Here's how the part is built. I have some questions about the finished solid (model axes, mm). Give positions to 0.01 mm unless a question says otherwise; leave off trailing zeros. Order: outer loops, then holes, each group sorted by start corner. A loop starts at its lowest first (then second) coordinate and runs counter-clockwise, first axis right, second up. Notation, with made-up numbers: (56, 53) -> (105, 53) arc R10 ccw to (105, 60) -> close; hole circle Ø3 at (28.25, 89). An arc over 180 degrees is marked (long way). Write each question's results on one line, items separated by ' | '. Start each with the question number.
Q1. Imagine slicing it at D-D, the plane x = -51. Please give me the cut outline in (y, z).
Q2. Imagine slicing it at B-B, the plane y = 6.5. Please give me the cut outline in (x, z).
Q3. I'm going to push flat-ended pins straight in: pin 1 (3 mm diameter, centred on x = 68.5, y = -68.5, fed in from +Z); pin 2 (1.2 mm diameter, centred on y = -42.5, z = 2, fed in from -X). Where does each tip first touch, or does it pass through?
Q4. Imagine slicing it at C-C, the plane z = 0.85. Please give me the cut outline in (x, y).
Q5. Imagine slicing it at A-A, the plane x = -68.5. Please give me the cut outline in (y, z).
Q6. I need wall thicknesses on line 1 along Y through (x, z) = (68.5, 2); line 2 along Y through (x, z) = (-3.5, 1.45); line 3 along X through (y, z) = (-68.5, 2). Which ranges of each line are inside material? Lowest first, please. Write a range as [from, to].
```python
from build123d import *

# Parameters (mm, degrees)
F1_DEPTH = 2.5
F2_R     = 1.75
F3_DEPTH = 3.5
F4_DEPTH = 1
F5_R     = 1


with BuildPart() as f1:
    # F0 (on Top) → F1 (new body)
    with BuildSketch(Plane.XY):
        Polygon((-10, -75), (75, -75), (75, 75), (-75, 75), (-75, 0), (-10, 0), align=None)
    extrude(amount=F1_DEPTH)

    # F2 (on face) → F3 (cut)
    with BuildSketch(Plane.XY.offset(2.5)):
        with Locations((-68.5, 68.5)):
            Circle(F2_R)
        with Locations((68.5, 68.5)):
            Circle(F2_R)
        with Locations((68.5, -68.5)):
            Circle(F2_R)
        with Locations((-3.5, -68.5)):
            Circle(F2_R)
        with Locations((-68.5, 6.5)):
            Circle(F2_R)
        with Locations((-3.5, -1.5)):
            Circle(F2_R)
    extrude(amount=-F3_DEPTH, mode=Mode.SUBTRACT)

    # F2 (on face) → F4 (join)
    with BuildSketch(Plane.XY.offset(2.5)):
        Polygon((73.5, 72.4), (-72.4, 72.4), (-72.4, 2.6), (-7.4, 2.6), (-7.4, -72.4), (72.4, -72.4), align=None)
        with Locations((-3.5, -68.5)):
            Circle(F2_R, mode=Mode.SUBTRACT)
        with Locations((-3.5, -1.5)):
            Circle(F2_R, mode=Mode.SUBTRACT)
        with Locations((68.5, -68.5)):
            Circle(F2_R, mode=Mode.SUBTRACT)
        with Locations((-68.5, 6.5)):
            Circle(F2_R, mode=Mode.SUBTRACT)
        with Locations((-68.5, 68.5)):
            Circle(F2_R, mode=Mode.SUBTRACT)
        with Locations((68.5, 68.5)):
            Circle(F2_R, mode=Mode.SUBTRACT)
    extrude(amount=F4_DEPTH)

    # F5
    f5_edges = [f1.edges().sort_by_distance(p)[0] for p in [
        (-10, 0, 1.25),
        (-10, -75, 1.25),
        (75, -75, 1.25),
        (75, 75, 1.25),
        (-75, 75, 1.25),
        (-75, 0, 1.25),
    ]]
    fillet(f5_edges, radius=F5_R)


solid = f1.part
```
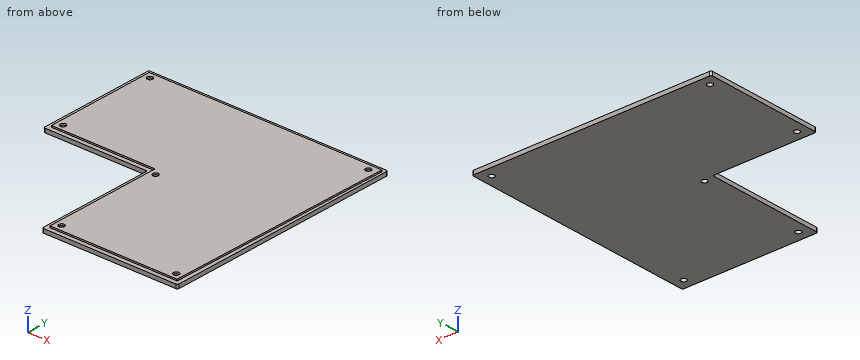
Geometry check:
1) outline: (0, 0) -> (75, 0) -> (75, 2.5) -> (72.4, 2.5) -> (72.4, 3.5) -> (2.6, 3.5) -> (2.6, 2.5) -> (0, 2.5) -> close
2) outline: (-75, 0) -> (-70.25, 0) -> (-70.25, 3.5) -> (-72.4, 3.5) -> (-72.4, 2.5) -> (-75, 2.5) -> close; (-66.75, 0) -> (75, 0) -> (75, 2.5) -> (73, 2.5) -> (73, 3.5) -> (-66.75, 3.5) -> close
3) pin 1: through | pin 2: x = -10
4) outline: (-75, 1) arc R1 ccw to (-74, 0) -> (-11, 0) arc R1 cw to (-10, -1) -> (-10, -74) arc R1 ccw to (-9, -75) -> (74, -75) arc R1 ccw to (75, -74) -> (75, 74) arc R1 ccw to (74, 75) -> (-74, 75) arc R1 ccw to (-75, 74) -> close; hole circle Ø3.5 at (-68.5, 6.5); hole circle Ø3.5 at (-68.5, 68.5); hole circle Ø3.5 at (-3.5, -68.5); hole circle Ø3.5 at (-3.5, -1.5); hole circle Ø3.5 at (68.5, -68.5); hole circle Ø3.5 at (68.5, 68.5)
5) outline: (0, 0) -> (4.75, 0) -> (4.75, 3.5) -> (2.6, 3.5) -> (2.6, 2.5) -> (0, 2.5) -> close; (8.25, 0) -> (66.75, 0) -> (66.75, 3.5) -> (8.25, 3.5) -> close; (70.25, 0) -> (75, 0) -> (75, 2.5) -> (72.4, 2.5) -> (72.4, 3.5) -> (70.25, 3.5) -> close
6) line 1: [-75, -70.25], [-66.75, 66.75], [70.25, 75] | line 2: [-75, -70.25], [-66.75, -3.25], [0.25, 75] | line 3: [-10, -5.25], [-1.75, 66.75], [70.25, 75]
